Check sheet for the modelled part. Datum: model origin and axes. Units: mm. A direction names the side the tool comes from. Round coordinates to 2 decimals unless told otherwise and drop trailing zeros. Loops run counter-clockwise (first coordinate to the right, second up) from the corner with the lowest first, then second, coordinate; pieces in that order, holes last. Notation, with made-up numbers: (-10, 84.5) -> (26, 84.5) arc R10 ccw to (26, 94.5) -> close; hole circle Ø5 at (21, 50.5). An arc over 180 degrees is marked (long way). One line per item, written item: value. Start each with the question number.
1. Cross-section at A-A on z = 6. Record the cut outline in (x, y), then the cut area to 3 significant figures.
2. Material ranges on L1, parallel to Y at x = 2, z = -0.5; L2, parallel to Y at x = -3, z = 8.5; L3, parallel to Z at x = 8, y = 7.5, recorded low to high.
3. Go/stop test with flat-tipped pins: pin 1 (3 mm diameter, centred on x = -4, z = 2.5, fed in from -Y); pin 2 (10 mm diameter, centred on x = -11, y = -12, fed in from -Z); pin 3 (4 mm diameter, centred on x = -15.84, y = 14.31, fed in from +Z); pin 4 (1.5 mm diameter, centred on y = -10, z = 4, fed in from -X). Record where each tip stops, or that it passes through.
4. Set-up check for faces 1 (the face through (6.8, -15, 1)), 2 (the face through (-16.991, 0, -1)), 3 (the face through (0, -11.5, -1)), 4 (the face through (16.991, 0, -1)): record each of +Z, -Z, +X, -X, +Y, -Y from which the full face is reachable in a straight line by a thin tool's end or side.
5. Cross-section at B-B on x = -4. Record the cut outline in (y, z), then the cut area to 3 significant figures.
6. Release check for a two-part mould opening along X. For faces 5 (the face through (-6.8, -15, 1)), 6 (the face through (0, 13, 0)), 7 (the face through (-17.8, 0, 1)) record: +X half, -X half, draft (parallel to the pull), parting line (faces both ways), or undercut.
7. Cross-section at C-C on y = 4.5. Record the cut outline in (x, z).
from build123d import *

# Parameters (mm, degrees)
SKETCH1_R           = 1.5
BOSS_EXTRUDE1_DEPTH = 1.4
SKETCH2_W           = 33.982309018
SKETCH2_H           = 23
BOSS_EXTRUDE2_DEPTH = 1.3
BOSS_EXTRUDE3_DEPTH = 8


with BuildPart() as part:
    # Sketch1 → Boss-Extrude1 (new body)
    with BuildSketch(Plane.XY):
        Polygon((17.8, 16.8), (-17.8, 16.8), (-17.8, -16.8), (-6.8, -16.8), (-6.8, -12.8), (6.8, -12.8), (6.8, -16.8), (17.8, -16.8), align=None)
        with Locations((-15.843700026, -14.313574824)):
            Circle(SKETCH1_R, mode=Mode.SUBTRACT)
        with Locations((15.843700026, -14.313574824)):
            Circle(SKETCH1_R, mode=Mode.SUBTRACT)
        with Locations((-15.843700026, 14.313574824)):
            Circle(SKETCH1_R, mode=Mode.SUBTRACT)
        with Locations((15.843700026, 14.313574824)):
            Circle(SKETCH1_R, mode=Mode.SUBTRACT)
    extrude(amount=BOSS_EXTRUDE1_DEPTH)

    # Sketch2 → Boss-Extrude2 (add)
    with BuildSketch(Plane(origin=(0, 0, 0), x_dir=(-1, 0, 0), z_dir=(0, 0, -1))):
        Rectangle(SKETCH2_W, SKETCH2_H)
    extrude(amount=BOSS_EXTRUDE2_DEPTH)

    # Sketch3 → Boss-Extrude3 (add)
    with BuildSketch(Plane.XY.offset(1.4)):
        Polygon((-0.625701938, 14.051390723), (-0.836940095, 14.417265944), (-1.259416409, 14.417265944), (-1.470654566, 14.051390723), (-1.259416409, 13.685515503), (-0.836940095, 13.685515503), align=None)
        Polygon((-2.625701938, 14.051390723), (-2.836940095, 14.417265944), (-3.259416409, 14.417265944), (-3.470654566, 14.051390723), (-3.259416409, 13.685515503), (-2.836940095, 13.685515503), align=None)
        Polygon((1.374298062, 14.051390723), (1.163059905, 14.417265944), (0.740583591, 14.417265944), (0.529345434, 14.051390723), (0.740583591, 13.685515503), (1.163059905, 13.685515503), align=None)
        Polygon((3.374298062, 14.051390723), (3.163059905, 14.417265944), (2.740583591, 14.417265944), (2.529345434, 14.051390723), (2.740583591, 13.685515503), (3.163059905, 13.685515503), align=None)
    extrude(amount=BOSS_EXTRUDE3_DEPTH)


solid = part.part
Taken from the geometry:
1. outline: (-3.47, 14.05) -> (-3.26, 13.69) -> (-2.84, 13.69) -> (-2.63, 14.05) -> (-2.84, 14.42) -> (-3.26, 14.42) -> close; (-1.47, 14.05) -> (-1.26, 13.69) -> (-0.84, 13.69) -> (-0.63, 14.05) -> (-0.84, 14.42) -> (-1.26, 14.42) -> close; (0.53, 14.05) -> (0.74, 13.69) -> (1.16, 13.69) -> (1.37, 14.05) -> (1.16, 14.42) -> (0.74, 14.42) -> close; (2.53, 14.05) -> (2.74, 13.69) -> (3.16, 13.69) -> (3.37, 14.05) -> (3.16, 14.42) -> (2.74, 14.42) -> close
1. area: 1.85 mm2
2. L1: y = -11.5 to 11.5
2. L2: y = 13.69 to 14.42
2. L3: z = -1.3 to 1.4
3. pin 1: stops at y = -12.8
3. pin 2: stops at z = -1.3
3. pin 3: stops at z = 1.4
3. pin 4: passes through
4. face 1: +Z, -Z, -Y
4. face 2: -Z, -X, +Y, -Y
4. face 3: -Z, +X, -X, -Y
4. face 4: -Z, +X, +Y, -Y
5. outline: (-12.8, 0) -> (-11.5, 0) -> (-11.5, -1.3) -> (11.5, -1.3) -> (11.5, 0) -> (16.8, 0) -> (16.8, 1.4) -> (-12.8, 1.4) -> close
5. area: 71.3 mm2
6. face 5: undercut
6. face 6: draft
6. face 7: -X half
7. outline: (-17.8, 0) -> (-16.99, 0) -> (-16.99, -1.3) -> (16.99, -1.3) -> (16.99, 0) -> (17.8, 0) -> (17.8, 1.4) -> (-17.8, 1.4) -> close
